Part print with two shaded views. Sizes in mm from the minimum x, y, z corner. A direction names the side the tool comes from. Round coordinates to 2 decimals unless told otherwise and drop trailing zeros. Loops run counter-clockwise (first coordinate to the right, second up) from the corner with the lowest first, then second, coordinate; pieces in that order, holes last. Notation, with made-up numbers: (83.25, 54) - (122.25, 54) arc R21 cw to (122.25, 92) - close; hole circle Ø4 at (68, 85.5). An arc over 180 degrees is marked (long way). Write each question's results on one line, items separated by ' | '. Start each with the question number.
(1) Mould opens along X. For the marked faces 5, 6 and 7 say: released by +X, released by -X, zero draft, split by the parting line, or undercut.
(2) Flat gauge pins, fed straight in: P1, Ø1, axis at x = 44.5, y = 16, coming from the +Z side; P2, Ø10, axis at x = 32.5, z = 24.5, coming from the +Y side; P3, Ø2, axis at y = 22, z = 5.5, coming from the -X side; P4, Ø5.5, axis at y = 12, z = 11.5, coming from the +X side. Where does each tip first touch, or does it go through?
(3) Cut at B-B, the plane x = 25. List the corners of the cut face in (y, z), then the cut area to 3 significant figures.
(4) Tool access for the marked faces 1, 2, 3 and 4: list every direction of +Z, -Z, +X, -X, +Y, -Y with a clear straight run to the whole face (end or side of a thin tool).
(5) Drill centre lines: L1, parallel to X at y = 12.5, z = 4.5 (1 decimal); L2, parallel to Y at x = 18, z = 22.5; L3, parallel to Z at x = 13, y = 24.5. Where is each one in solid material? Low to high.
(6) Cut at C-C, the plane z = 30.5. List the corners of the cut face in (x, y) (1 decimal), then the cut area to 3 significant figures.
(7) Cut at D-D, the plane z = 11. List the corners of the cut face in (x, y) (1 decimal), then the cut area to 3 significant figures.
(8) Cut at A-A, the plane y = 27.94. List the corners of the cut face in (x, z) (1 decimal).
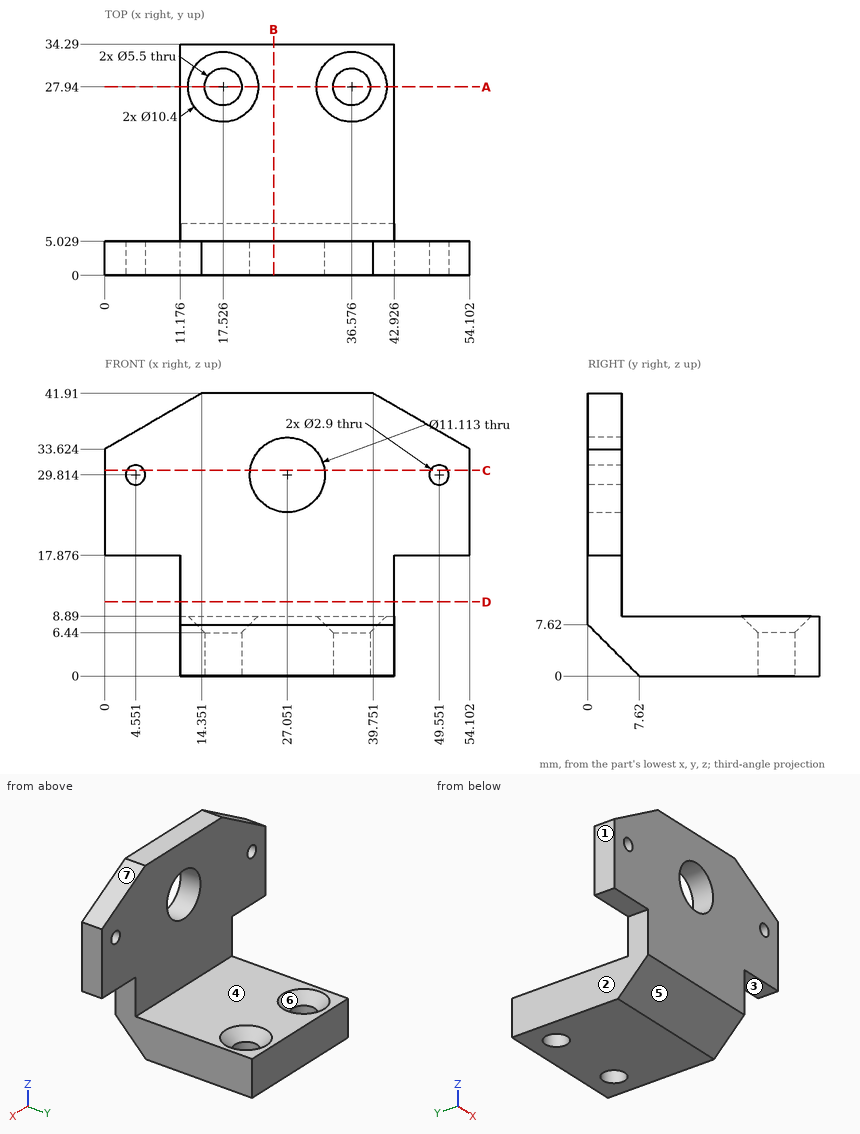
A:
1) face 5: zero draft | face 6: undercut | face 7: released by +X
2) P1: through | P2: y = 5.03 | P3: x = 11.18 | P4: x = 42.93
3) outline: (0, 7.62) - (7.62, 0) - (34.29, 0) - (34.29, 8.89) - (5.03, 8.89) - (5.03, 24.65) - (0, 24.65) - close; (0, 34.98) - (5.03, 34.98) - (5.03, 41.91) - (0, 41.91) - close | area: 390 mm2
4) face 1: +Z, -Z, -X, +Y, -Y | face 2: -Z, -X, +Y, -Y | face 3: -Z, +X, +Y, -Y | face 4: +Z, +X, -X, +Y
5) L1: 11.2 to 42.9 | L2: 0 to 5.03 | L3: 0 to 8.89
6) outline: (0, 0) - (3.3, 0) - (3.3, 5) - (0, 5) - close; (5.8, 0) - (21.5, 0) - (21.5, 5) - (5.8, 5) - close; (32.6, 0) - (48.3, 0) - (48.3, 5) - (32.6, 5) - close; (50.8, 0) - (54.1, 0) - (54.1, 5) - (50.8, 5) - close | area: 191 mm2
7) outline: (11.2, 0) - (42.9, 0) - (42.9, 5) - (11.2, 5) - close | area: 160 mm2
8) outline: (11.2, 0) - (14.8, 0) - (14.8, 6.4) - (12.3, 8.9) - (11.2, 8.9) - close; (20.3, 0) - (33.8, 0) - (33.8, 6.4) - (31.4, 8.9) - (22.7, 8.9) - (20.3, 6.4) - close; (39.3, 0) - (42.9, 0) - (42.9, 8.9) - (41.8, 8.9) - (39.3, 6.4) - close
